Source: three-view drawing plus pictorial views. Frame: mm from the lowest corner of the part. Give positions to 0.01 mm unless a question says otherwise; leave off trailing zeros. Order: outer loops, then holes, each group sorted by start corner. A loop starts at its lowest first (then second) coordinate and runs counter-clockwise, first axis right, second up.
1) First-contact query: P1, Ø1, axis at x = 45, y = 1, coming from the -Z side; P2, Ø1, axis at y = 2, z = 8, coming from the +X side; P3, Ø1, axis at x = 41, y = 0.5, coming from the +Z side. Flat tips, straight axial feed; report the tip coordinate or a pass-through.
2) Section B-B, the plane x = 25. Return loops of the section in (y, z).
3) Section C-C, the plane z = 25. Return loops of the section in (x, y), plus the area to 3 significant figures.
4) Section D-D, the plane y = 0.7. Give the number of separate pieces and of enclosed holes in the cut face, plus the area to 3 significant figures.
5) Material intervals for line 1 (X direction, y = 0.5, z = 25); line 2 (X direction, y = 1.3, z = 41.5); line 3 (Z direction, x = 25.5, y = 0.95), sorted ascending.
6) Section A-A, the plane z = 41.5. Return loops of the section in (x, y).
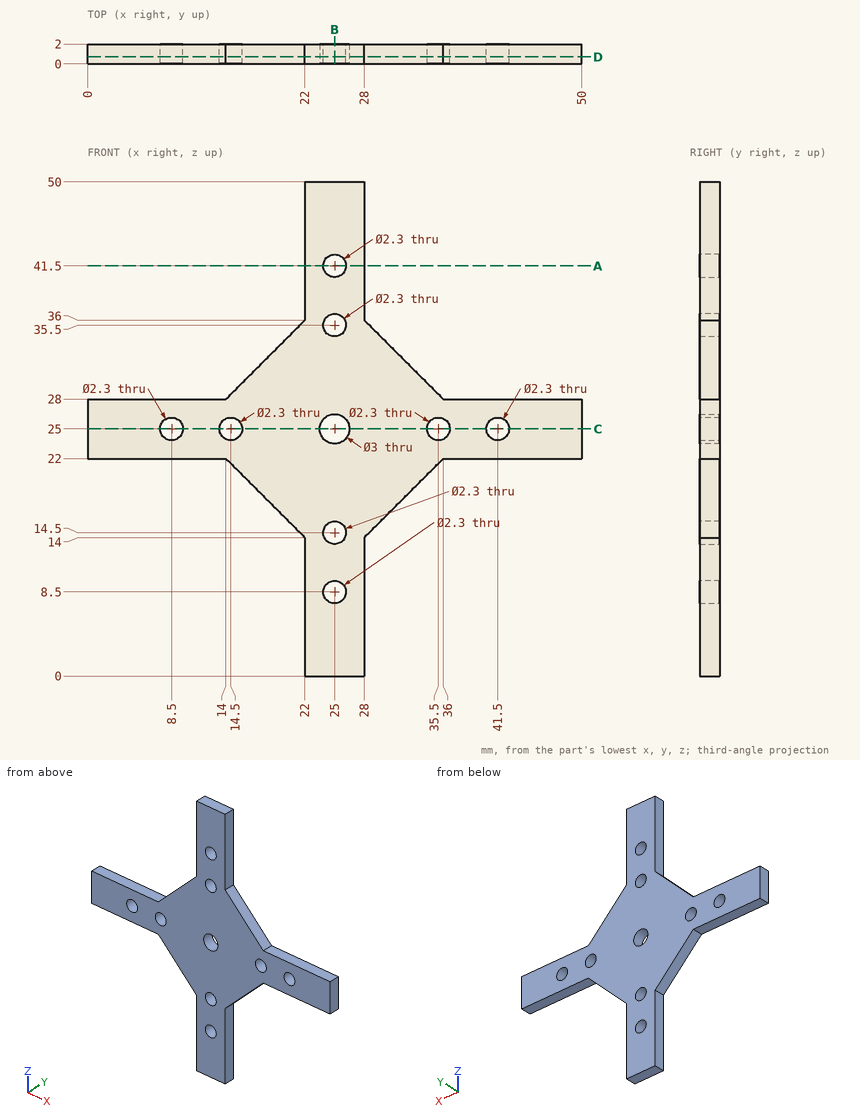
From the geometry:
1. P1: stops at z = 22
1. P2: stops at x = 28
1. P3: stops at z = 28
2. outline: (0, 0) - (2, 0) - (2, 7.35) - (0, 7.35) - close; (0, 9.65) - (2, 9.65) - (2, 13.35) - (0, 13.35) - close; (0, 15.65) - (2, 15.65) - (2, 23.5) - (0, 23.5) - close; (0, 26.5) - (2, 26.5) - (2, 34.35) - (0, 34.35) - close; (0, 36.65) - (2, 36.65) - (2, 40.35) - (0, 40.35) - close; (0, 42.65) - (2, 42.65) - (2, 50) - (0, 50) - close
3. outline: (0, 0) - (7.35, 0) - (7.35, 2) - (0, 2) - close; (9.65, 0) - (13.35, 0) - (13.35, 2) - (9.65, 2) - close; (15.65, 0) - (23.5, 0) - (23.5, 2) - (15.65, 2) - close; (26.5, 0) - (34.35, 0) - (34.35, 2) - (26.5, 2) - close; (36.65, 0) - (40.35, 0) - (40.35, 2) - (36.65, 2) - close; (42.65, 0) - (50, 0) - (50, 2) - (42.65, 2) - close
3. area: 75.6 mm2
4. separate pieces: 1
4. enclosed holes: 9
4. area: 652 mm2
5. line 1: x = 0 to 7.35, 9.65 to 13.35, 15.65 to 23.5, 26.5 to 34.35, 36.65 to 40.35, 42.65 to 50
5. line 2: x = 22 to 23.85, 26.15 to 28
5. line 3: z = 0 to 7.46, 9.54 to 13.46, 15.54 to 23.59, 26.41 to 34.46, 36.54 to 40.46, 42.54 to 50
6. outline: (22, 0) - (23.85, 0) - (23.85, 2) - (22, 2) - close; (26.15, 0) - (28, 0) - (28, 2) - (26.15, 2) - close
